from build123d import *

# Parameters (mm, degrees)
BOSS_EXTRUDE1_DEPTH = 50
CUT_EXTRUDE1_START  = -15
CUT_EXTRUDE1_DEPTH  = 165
SKETCH3_R           = 15
BOSS_EXTRUDE2_DEPTH = 5
SKETCH4_R           = 16
BOSS_EXTRUDE3_DEPTH = 5
SKETCH5_R           = 10
CUT_EXTRUDE2_DEPTH  = 251.249875125
FILLET1_R           = 5
HOLE1_D             = 5
HOLE1_DEPTH         = 40
HOLE1_CBORE_D       = 6
HOLE1_CBORE_DEPTH   = 10
HOLE1_TIP           = 1.502151548
HOLE2_D             = 3
HOLE2_CSINK_D       = 5
HOLE2_CSINK_ANGLE   = 90
HOLE4_D             = 3
HOLE4_CSINK_D       = 5
HOLE4_CSINK_ANGLE   = 90
BOSS_EXTRUDE7_DEPTH = 20
BOSS_EXTRUDE9_DEPTH = 3


with BuildPart() as part:
    # Sketch1 → Boss-Extrude1 (new, symmetric)
    with BuildSketch(Plane.XY):
        with BuildLine():
            Line((0, 0), (220, 0))
            Line((220, 0), (220, 75))
            ThreePointArc((220, 75), (217.071067812, 82.071067812), (210, 85))
            Line((210, 85), (185, 85))
            Line((185, 85), (185, 60))
            Line((185, 60), (180, 60))
            Line((180, 60), (180, 57))
            Line((180, 57), (0, 57))
            Line((0, 57), (0, 0))
        make_face()
    extrude(amount=BOSS_EXTRUDE1_DEPTH, both=True)

    # Sketch2 → Cut-Extrude1 (cut)
    with BuildSketch(Plane.ZY.offset(CUT_EXTRUDE1_START)):
        Polygon((-30, 0), (-30, 10), (-26, 10), (-26, 13), (-20, 13), (-20, 57), (20, 57), (20, 13), (26, 13), (26, 10), (30, 10), (30, 0), align=None)
    extrude(amount=-CUT_EXTRUDE1_DEPTH, mode=Mode.SUBTRACT)

    # Sketch3 → Boss-Extrude2 (add)
    with BuildSketch(Plane.ZY):
        with Locations(Location((0, 30, 0), (0, 0, 270))):
            Circle(SKETCH3_R)
    extrude(amount=BOSS_EXTRUDE2_DEPTH)

    # Sketch4 → Boss-Extrude3 (add)
    with BuildSketch(Plane(origin=(220, 0, 0), x_dir=(0, 0, -1), z_dir=(1, 0, 0))):
        with Locations(Location((0, 30, 0), (0, 0, 180))):
            Circle(SKETCH4_R)
    extrude(amount=BOSS_EXTRUDE3_DEPTH)

    # Sketch5 → Cut-Extrude2 (cut, through all)
    with BuildSketch(Plane(origin=(225, 0, 0), x_dir=(0, 0, -1), z_dir=(1, 0, 0))):
        with Locations((0, 30)):
            Circle(SKETCH5_R)
    extrude(amount=-CUT_EXTRUDE2_DEPTH, mode=Mode.SUBTRACT)

    # Fillet1
    fillet1_edges = [part.edges().sort_by_distance(p)[0] for p in [
        (0, 45, 0),
        (220, 30, -16),
    ]]
    fillet(fillet1_edges, radius=FILLET1_R - 0.0001)  # a hair under: the kernel refuses the full size

    # Hole1
    with Locations(Plane(origin=(185, 72.5, -30), x_dir=(0, 0, -1), z_dir=(-1, 0, 0))):
        with Locations((0, 0), (-60, 0)):
            CounterBoreHole(HOLE1_D / 2, HOLE1_CBORE_D / 2, HOLE1_CBORE_DEPTH, depth=HOLE1_DEPTH)
            with Locations((0, 0, -(HOLE1_DEPTH + HOLE1_TIP / 2))):  # 118° drill point
                Cone(0, HOLE1_D / 2, HOLE1_TIP, mode=Mode.SUBTRACT)

    # Hole2 (through all)
    with Locations(Plane(origin=(205, 85, 0), x_dir=(0, 0, 1), z_dir=(0, 1, 0))):
        with Locations((0, 0)):
            CounterSinkHole(HOLE2_D / 2, HOLE2_CSINK_D / 2, counter_sink_angle=HOLE2_CSINK_ANGLE)

    # Hole4 (through all)
    with Locations(Plane(origin=(5, 57, 0), x_dir=(1, 0, 0), z_dir=(0, 1, 0))):
        with Locations((0, 0)):
            CounterSinkHole(HOLE4_D / 2, HOLE4_CSINK_D / 2, counter_sink_angle=HOLE4_CSINK_ANGLE)

    # Sketch18 → Boss-Extrude7 (add)
    with BuildSketch(Plane.XZ):
        with BuildLine():
            Line((55, 50), (95, 94.291635381))
            Line((95, 94.291635381), (107, 94.291635381))
            Line((107, 94.291635381), (107, 81.291635381))
            ThreePointArc((107, 81.291635381), (115, 73.291635381), (123, 81.291635381))
            Line((123, 81.291635381), (123, 94.291635381))
            Line((123, 94.291635381), (135, 94.291635381))
            Line((135, 94.291635381), (175, 50))
            Line((175, 50), (55, 50))
        make_face()
    boss_extrude7 = extrude(amount=-BOSS_EXTRUDE7_DEPTH)

    # Mirror4: Boss-Extrude7 across plane
    add(boss_extrude7.mirror(Plane.XY))

    # Sketch21 → Boss-Extrude9 (add)
    with BuildSketch(Plane(origin=(0, 20, 0), x_dir=(1, 0, 0), z_dir=(0, 1, 0))):
        with BuildLine():
            Line((128, 94.291635381), (128, 81.291635381))
            ThreePointArc((128, 81.291635381), (115, 68.291635381), (102, 81.291635381))
            Line((102, 81.291635381), (102, 94.291635381))
            Line((102, 94.291635381), (107, 94.291635381))
            Line((107, 94.291635381), (107, 81.291635381))
            ThreePointArc((107, 81.291635381), (115, 73.291635381), (123, 81.291635381))
            Line((123, 81.291635381), (123, 94.291635381))
            Line((123, 94.291635381), (128, 94.291635381))
        make_face()
    boss_extrude9 = extrude(amount=BOSS_EXTRUDE9_DEPTH)

    # Mirror5: Boss-Extrude9 across plane
    add(boss_extrude9.mirror(Plane.XY))


solid = part.part
Input: part model. Units: mm. Frame: model coordinates. A direction names the side the tool comes from. Give positions to 0.01 mm unless a question says otherwise; leave off trailing zeros. Write each loop counter-clockwise with the first axis right and the second up, starting at its lowest first coordinate (ties: lowest second). Pieces come first, ordered by that corner, then holes. Notation, with made-up numbers: M 10.25,-28.5 L 64.25,-28.5 A37 ccw 64.25,7.5 Z; hole C 43.5,57.5 d1. An arc over 180 degrees is marked long. Use one line per item in the form item = value.
1. Ray query, L1, parallel to Z at x = 27, y = 14.5; L2, parallel to X at y = 11, z = -16; L3, parallel to Z at x = 208, y = 72. Return the intervals inside material, ascending.
Outcome:
L1 = -50 to -20, 20 to 50
L2 = 0 to 15, 180 to 220
L3 = -50 to -32.45, -27.55 to 27.55, 32.45 to 50
2. Cut plane C-C on x = 82. Return loops of the section in (y, z).
Outcome:
outline = M 0,-79.9 L 20,-79.9 L 20,-50 L 57,-50 L 57,-20 L 13,-20 L 13,-26 L 10,-26 L 10,-30 L 0,-30 Z; M 0,30 L 10,30 L 10,26 L 13,26 L 13,20 L 57,20 L 57,50 L 20,50 L 20,79.9 L 0,79.9 Z
3. Reachability of faces 5 (the face through (185, 73, 1)), 6 (the face through (96, 35, 20)), 7 (the face through (195, 70, -29)), 8 (the face through (121, 23, 75.7)), 9 (the face through (114.824, 11.339, -73.294)) from +Z, -Z, +X, -X, +Y, -Y: full face, straight path, thin tool, end or side. Return the list, or none.
Outcome:
face_5 = +Z, -Z, -X, +Y
face_6 = +Y, -Y
face_7 = -X
face_8 = +Z, +X, -X, +Y
face_9 = -Z, +Y, -Y
4. First-contact query: P1, Ø1, axis at x = 169.5, z = 47.5, coming from the +Y side; P2, Ø2.5, axis at x = 183, z = 0.5, coming from the +Y side; P3, Ø10, axis at x = 80, y = 42.5, coming from the -Z side; P4, Ø13, axis at x = 132, y = 27.5, coming from the +Z side. Flat tips, straight axial feed; report the tip coordinate or a pass-through.
Outcome:
P1 = 57
P2 = 60
P3 = -50
P4 = 94.29
5. Cut plane A-A on y = 72.5. Return loops of the section in (x, z).
Outcome:
outline = M 185,-50 L 220,-50 L 220,-32.5 L 195,-32.5 L 195,-33 L 185,-33 Z; M 185,-27 L 195,-27 L 195,-27.5 L 220,-27.5 L 220,27.5 L 195,27.5 L 195,27 L 185,27 Z; M 185,33 L 195,33 L 195,32.5 L 220,32.5 L 220,50 L 185,50 Z; hole C 205,0 d3
6. Cut plane D-D on z = 46.5. Return loops of the section in (x, y).
Outcome:
outline = M 0,0 L 220,0 L 220,75 A10 ccw 210,85 L 185,85 L 185,60 L 180,60 L 180,57 L 0,57 Z
7. Mould query, pull axis Z, two halves, no side actions, for faces 1 (the face through (129, 11, 94.292)), 2 (the face through (123, 11, 88)), 3 (the face through (115.286, 21.479, -68.295)), 4 (the face through (96, 13, 23)). Classes: released by +Z, released by -Z, zero draft, split by the parting line, or undercut.
Outcome:
face_1 = released by +Z
face_2 = zero draft
face_3 = undercut
face_4 = undercut
